```python
from build123d import *

# Parameters (mm, degrees)
SKETCH1_R           = 7
SKETCH1_R_2         = 4
BOSS_EXTRUDE1_DEPTH = 4
CHAMFER1_SIZE       = 0.2
FILLET1_R           = 0.5


with BuildPart() as part:
    # Sketch1 → Boss-Extrude1 (new body)
    with BuildSketch(Plane(origin=(0, 0, 0), x_dir=(1, 0, 0), z_dir=(0, 1, 0))):
        Circle(SKETCH1_R)
        Circle(SKETCH1_R_2, mode=Mode.SUBTRACT)
    extrude(amount=BOSS_EXTRUDE1_DEPTH)

    # Chamfer1
    chamfer1_edges = [part.edges().sort_by_distance(p)[0] for p in [
        (-4, 0, 0),
        (-4, 4, 0),
    ]]
    chamfer(chamfer1_edges, length=CHAMFER1_SIZE)

    # Fillet1
    fillet1_edges = [part.edges().sort_by_distance(p)[0] for p in [
        (-7, 0, 0),
        (-7, 4, 0),
    ]]
    fillet(fillet1_edges, radius=FILLET1_R)


solid = part.part
```
The listing builds one solid part. Answer for the finished solid, in the listing's coordinates (mm). Give positions to 0.01 mm unless a question says otherwise; leave off trailing zeros. Loops run counter-clockwise (first coordinate to the right, second up) from the corner with the lowest first, then second, coordinate; pieces in that order, holes last. Notation, with made-up numbers: M 40,11.25 L 71,11.25 A13 cw 71,21.25 Z; hole C 13.25,43 d7. An arc over 180 degrees is marked long. One line per item, written item: value.
1. Find the intervals of material crossed by probe 1 along X at (y, z) = (2.35, 0); probe 2 along X at (y, z) = (0.6, 3.25), in increasing order.
Found:
probe 1: -7 to -4, 4 to 7
probe 2: -6.2 to -2.33, 2.33 to 6.2
2. Section B-B on z = 0 is taken. Determine the outline of the cut face in (x, y).
Found:
outline: M -7,0.5 A0.5 ccw -6.5,0 L -4.2,0 L -4,0.2 L -4,3.8 L -4.2,4 L -6.5,4 A0.5 ccw -7,3.5 Z; M 4,0.2 L 4.2,0 L 6.5,0 A0.5 ccw 7,0.5 L 7,3.5 A0.5 ccw 6.5,4 L 4.2,4 L 4,3.8 Z
3. Section C-C on y = 1.65 is taken. Determine the outline of the cut face in (x, z), plus the area to 3 significant figures.
Found:
outline: C 0,0 d14; hole C 0,0 d8
area: 104 mm^2
4. For a pull along Z with two mould halves and no side action, classify faces 1 (the face through (1.4, 4, 4.2)), 2 (the face through (6.466, 1.979, 2.681)), 3 (the face through (-0.867, 1.975, 3.905)) as pulls with the +Z half, pulls with the -Z half, needs draft (parallel to the pull), parting line crosses it, or undercut.
Found:
face 1: needs draft
face 2: parting line crosses it
face 3: undercut
5. Section A-A on x = 0 is taken. Determine the outline of the cut face in (y, z), plus the area to 3 significant figures.
Found:
outline: M 0,-6.5 A0.5 ccw 0.5,-7 L 3.5,-7 A0.5 ccw 4,-6.5 L 4,-4.2 L 3.8,-4 L 0.2,-4 L 0,-4.2 Z; M 0,4.2 L 0.2,4 L 3.8,4 L 4,4.2 L 4,6.5 A0.5 ccw 3.5,7 L 0.5,7 A0.5 ccw 0,6.5 Z
area: 23.7 mm^2
